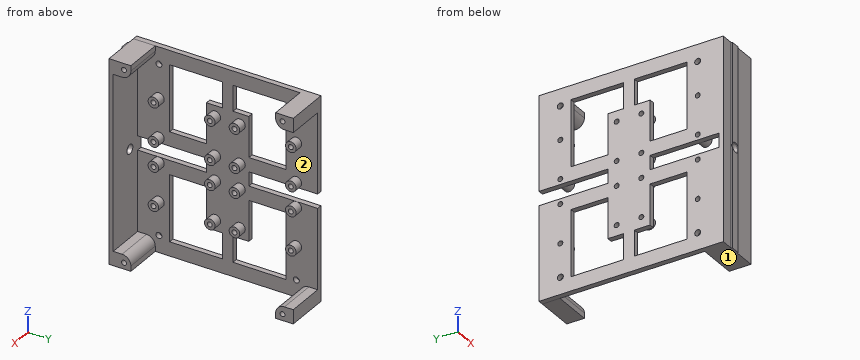
from build123d import *

# Parameters (mm, degrees)
SKETCH017_R          = 1.7
SKETCH017_W          = 39.1
SKETCH017_H          = 8
PAD006_DEPTH         = 3
SKETCH018_R          = 3
PAD007_DEPTH         = 5
SKETCH020_R          = 1.4
POCKET011_DEPTH      = 8.001
PAD008_DEPTH         = 22
SKETCH021_R          = 1.4
POCKET012_DEPTH      = 9
PAD009_DEPTH         = 115.2
SKETCH023_R          = 2.7
POCKET013_DEPTH      = 0.601
POCKET013_DEPTH_BACK = 104.601


with BuildPart() as part:
    # Sketch017 → Pad006 (new body)
    with BuildSketch(Plane.YZ):
        Polygon((0, 117.6), (104.6, 117.6), (104.6, 64), (65.5, 64), (65.5, 56), (104.6, 56), (104.6, 2.4), (0, 2.4), align=None)
        with Locations((14.5, 108)):
            Circle(SKETCH017_R, mode=Mode.SUBTRACT)
        with Locations((92.5, 108)):
            Circle(SKETCH017_R, mode=Mode.SUBTRACT)
        with Locations((92.5, 12)):
            Circle(SKETCH017_R, mode=Mode.SUBTRACT)
        with Locations((14.5, 12)):
            Circle(SKETCH017_R, mode=Mode.SUBTRACT)
        with Locations((21.95, 60)):
            Rectangle(SKETCH017_W, SKETCH017_H, mode=Mode.SUBTRACT)
        Polygon((86.5, 109.6), (86.5, 72), (65.5, 72), (65.5, 95), (56.5, 95), (56.5, 109.6), align=None, mode=Mode.SUBTRACT)
        Polygon((20.5, 72), (20.5, 109.6), (50.5, 109.6), (50.5, 95), (41.5, 95), (41.5, 72), align=None, mode=Mode.SUBTRACT)
        Polygon((86.5, 48), (86.5, 10.4), (56.5, 10.4), (56.5, 25), (65.5, 25), (65.5, 48), align=None, mode=Mode.SUBTRACT)
        Polygon((20.5, 10.4), (20.5, 48), (41.5, 48), (41.5, 25), (50.5, 25), (50.5, 10.4), align=None, mode=Mode.SUBTRACT)
    extrude(amount=PAD006_DEPTH)

    # Sketch018 → Pad007 (join)
    with BuildSketch(Plane.YZ.offset(3)):
        with Locations((14.5, 89)):
            Circle(SKETCH018_R)
        with Locations((46.5, 89)):
            Circle(SKETCH018_R)
        with Locations((60.5, 89)):
            Circle(SKETCH018_R)
        with Locations((92.5, 89)):
            Circle(SKETCH018_R)
        with Locations((92.5, 67)):
            Circle(SKETCH018_R)
        with Locations((60.5, 67)):
            Circle(SKETCH018_R)
        with Locations((46.5, 67)):
            Circle(SKETCH018_R)
        with Locations((14.5, 67)):
            Circle(SKETCH018_R)
        with Locations((14.5, 53)):
            Circle(SKETCH018_R)
        with Locations((46.5, 53)):
            Circle(SKETCH018_R)
        with Locations((60.5, 53)):
            Circle(SKETCH018_R)
        with Locations((92.5, 53)):
            Circle(SKETCH018_R)
        with Locations((92.5, 31)):
            Circle(SKETCH018_R)
        with Locations((60.5, 31)):
            Circle(SKETCH018_R)
        with Locations((46.5, 31)):
            Circle(SKETCH018_R)
        with Locations((14.5, 31)):
            Circle(SKETCH018_R)
    extrude(amount=PAD007_DEPTH)

    # Sketch020 → Pocket011 (cut, through all)
    with BuildSketch(Plane.YZ.offset(8)):
        with Locations((14.5, 89)):
            Circle(SKETCH020_R)
        with Locations((46.5, 89)):
            Circle(SKETCH020_R)
        with Locations((60.5, 89)):
            Circle(SKETCH020_R)
        with Locations((92.5, 89)):
            Circle(SKETCH020_R)
        with Locations((92.5, 67)):
            Circle(SKETCH020_R)
        with Locations((60.5, 67)):
            Circle(SKETCH020_R)
        with Locations((46.5, 67)):
            Circle(SKETCH020_R)
        with Locations((14.5, 67)):
            Circle(SKETCH020_R)
        with Locations((14.5, 53)):
            Circle(SKETCH020_R)
        with Locations((46.5, 53)):
            Circle(SKETCH020_R)
        with Locations((60.5, 53)):
            Circle(SKETCH020_R)
        with Locations((92.5, 53)):
            Circle(SKETCH020_R)
        with Locations((92.5, 31)):
            Circle(SKETCH020_R)
        with Locations((60.5, 31)):
            Circle(SKETCH020_R)
        with Locations((46.5, 31)):
            Circle(SKETCH020_R)
        with Locations((14.5, 31)):
            Circle(SKETCH020_R)
    extrude(amount=-POCKET011_DEPTH, mode=Mode.SUBTRACT)

    # Sketch019 → Pad008 (join)
    with BuildSketch(Plane.YZ.offset(3)):
        with BuildLine():
            ThreePointArc((94.6, 114.599982), (96.064466, 111.064448), (99.6, 109.599982))
            Line((104.6, 109.599982), (99.6, 109.599982))
            Line((104.6, 117.6), (104.6, 109.599982))
            Line((94.6, 117.6), (104.6, 117.6))
            Line((94.6, 114.599982), (94.6, 117.6))
        make_face()
        with BuildLine():
            ThreePointArc((99.6, 10.400018), (96.064473, 8.935559), (94.6, 5.400037))
            Line((94.6, 2.400018), (94.6, 5.400037))
            Line((104.6, 2.400018), (94.6, 2.400018))
            Line((104.6, 10.400018), (104.6, 2.400018))
            Line((99.6, 10.400018), (104.6, 10.400018))
        make_face()
        with BuildLine():
            ThreePointArc((7.4, 109.599982), (10.935527, 111.064441), (12.4, 114.599963))
            Line((12.4, 117.599982), (12.4, 114.599963))
            Line((0, 117.599982), (12.4, 117.599982))
            Line((0, 2.4), (0, 117.599982))
            Line((12.4, 2.4), (0, 2.4))
            Line((12.4, 5.400018), (12.4, 2.4))
            ThreePointArc((12.4, 5.400018), (10.935534, 8.935552), (7.4, 10.400018))
            Line((2.4, 10.400018), (7.4, 10.400018))
            Line((2.4, 109.599982), (2.4, 10.400018))
            Line((7.4, 109.599982), (2.4, 109.599982))
        make_face()
    extrude(amount=PAD008_DEPTH)

    # Sketch021 → Pocket012 (cut)
    with BuildSketch(Plane.YZ.offset(25)):
        with Locations((8.5, 114)):
            Circle(SKETCH021_R)
        with Locations((98.5, 114)):
            Circle(SKETCH021_R)
        with Locations((98.5, 6)):
            Circle(SKETCH021_R)
        with Locations((8.5, 6)):
            Circle(SKETCH021_R)
    extrude(amount=-POCKET012_DEPTH, mode=Mode.SUBTRACT)

    # Sketch022 → Pad009 (join)
    with BuildSketch(Plane.XY.offset(2.4)):
        Polygon((7, 0), (13, 0), (12.4, -0.6), (7.6, -0.6), align=None)
    extrude(amount=PAD009_DEPTH)

    # Sketch023 → Pocket013 (cut, two sides)
    with BuildSketch(Plane.XZ) as pocket013_sk:
        with Locations((10, 60)):
            Circle(SKETCH023_R)
    extrude(amount=POCKET013_DEPTH, mode=Mode.SUBTRACT)
    extrude(pocket013_sk.sketch, amount=-POCKET013_DEPTH_BACK, mode=Mode.SUBTRACT)


solid = part.part
CAD build for the part. Positions are in the model's coordinates, mm. Face numbers are marked on the shaded views. Give positions to 0.01 mm unless a question says otherwise; leave off trailing zeros. Write each loop counter-clockwise with the first axis right and the second up, starting at its lowest first coordinate (ties: lowest second). Pieces come first, ordered by that corner, then holes. Notation, with made-up numbers: (73, 72.25) -> (107, 72.25) arc R20 cw to (107, 79.25) -> close; hole circle Ø9 at (18.25, 4). An arc over 180 degrees is marked (long way). Return JSON: item names as keys, results as strings.
Item 1: Two-plate mould, pull along Y, no slides. Class the marked faces 1 and 2: +Y half, -Y half, draft (parallel to the pull), parting line (faces both ways), or undercut.
Answer below:
{"face 1": "draft", "face 2": "undercut"}
Item 2: Band-saw the part on B-B (y = 70.5). List the corners of the cut face in (x, z), then the cut area to 3 significant figures.
Answer below:
{"outline": "(0, 2.4) -> (3, 2.4) -> (3, 10.4) -> (0, 10.4) -> close; (0, 48) -> (3, 48) -> (3, 56) -> (0, 56) -> close; (0, 64) -> (3, 64) -> (3, 72) -> (0, 72) -> close; (0, 109.6) -> (3, 109.6) -> (3, 117.6) -> (0, 117.6) -> close", "area": "96.0 mm2"}
Item 3: Drop flat-ended pins along their axis: pin 1 (5 mm diameter, centred on x = 17, z = 20, fed in from +Y); pin 2 (3.5 mm diameter, centred on y = 8.5, z = 114, fed in from +X); pin 3 (12 mm diameter, centred on y = 88, z = 77.5, fed in from +X); pin 4 (3 mm diameter, centred on y = 92.5, z = 89, fed in from +X). Give the stop position or say it passes through.
Answer below:
{"pin 1": "stops at y = 2.4", "pin 2": "stops at x = 25", "pin 3": "stops at x = 3", "pin 4": "stops at x = 8"}
Item 4: Band-saw the part on D-D (x = 5). Give the number of separate pieces and of enclosed holes in the cut face, then the cut area to 3 significant figures.
Answer below:
{"separate pieces": "19", "enclosed holes": "16", "area": "929 mm2"}
Item 5: Drill centre lines: probe 1 along Z at (x, y) = (1.25, 36); probe 2 along X at (y, z) = (6.5, 48.5); probe 3 along Y at (x, z) = (23.25, 95). Where is each one in solid material? Low to high.
Answer below:
{"probe 1": "z = 2.4 to 10.4, 48 to 56, 64 to 72, 109.6 to 117.6", "probe 2": "x = 0 to 3", "probe 3": "y = 0 to 2.4"}
Item 6: Band-saw the part on C-C (z = 22.5). List the corners of the cut face in (x, y), then the cut area to 3 significant figures.
Answer below:
{"outline": "(0, 0) -> (7, 0) -> (7.6, -0.6) -> (12.4, -0.6) -> (13, 0) -> (25, 0) -> (25, 2.4) -> (3, 2.4) -> (3, 20.5) -> (0, 20.5) -> close; (0, 50.5) -> (3, 50.5) -> (3, 56.5) -> (0, 56.5) -> close; (0, 86.5) -> (3, 86.5) -> (3, 104.6) -> (0, 104.6) -> close", "area": "190 mm2"}
Item 7: Band-saw the part on A-A (x = 17.75). List the corners of the cut face in (y, z), then the cut area to 3 significant figures.
Answer below:
{"outline": "(0, 2.4) -> (12.4, 2.4) -> (12.4, 5.4) arc R5 ccw to (7.4, 10.4) -> (2.4, 10.4) -> (2.4, 109.6) -> (7.4, 109.6) arc R5 ccw to (12.4, 114.6) -> (12.4, 117.6) -> (0, 117.6) -> close; (94.6, 2.4) -> (104.6, 2.4) -> (104.6, 10.4) -> (99.6, 10.4) arc R5 ccw to (94.6, 5.4) -> close; (94.6, 114.6) arc R5 ccw to (99.6, 109.6) -> (104.6, 109.6) -> (104.6, 117.6) -> (94.6, 117.6) -> close; hole circle Ø2.8 at (8.5, 6); hole circle Ø2.8 at (8.5, 114); hole circle Ø2.8 at (98.5, 6); hole circle Ø2.8 at (98.5, 114)", "area": "550 mm2"}
